Model file for the job. Use its own axes, mm. A direction names the side the tool comes from. Round coordinates to 2 decimals unless told otherwise and drop trailing zeros. Loops run counter-clockwise (first coordinate to the right, second up) from the corner with the lowest first, then second, coordinate; pieces in that order, holes last. Notation, with made-up numbers: M 18,47 L 48,47 A33 ccw 48,83 Z; hole C 81.5,14 d11. An arc over 180 degrees is marked long. Use a Markdown table: item, result. Add a question column.
Q1. Cut at D-D (z = -72.9). Give the cut face in (x, y), plus the area to 3 significant figures.
Q2. Tool access for faces 1 (the face through (43, 2.8, -34)), 2 (the face through (8.8, 2, -61)), 3 (the face through (38, 3, -71)), 4 (the face through (45, 2, -56)), 5 (the face through (26.2, 2, -73)): list every direction of +Z, -Z, +X, -X, +Y, -Y with a clear straight run to the whole face (end or side of a thin tool).
Q3. Cut at A-A (x = 37.5). Give the cut face in (y, z).
Q4. Pin check, flat tips, straight feed: pin 1 (0.8 mm diameter, centred on y = 2, z = -44, fed in from +X); pin 2 (1.5 mm diameter, centred on y = 1.5, z = -58.5, fed in from +X); pin 3 (2 mm diameter, centred on y = 1.5, z = -20.5, fed in from -X). Stop position of each tip, or through.
Q5. Probe line 1 (X direction, y = 0.85, z = -50); line 2 (Z direction, x = 25, y = 1.1); line 3 (Z direction, x = 8, y = 2.85). List the from-to ranges inside material, lowest first. Write a range as from..to.
Q6. Cut at C-C (x = 21). Give the cut face in (y, z), plus the area to 3 significant figures.
Q7. Cut at B-B (z = -44). Give the cut face in (x, y).
Q8. Mould opens along Z. For faces 6 (the face through (-3, 2, -17)), 7 (the face through (2, 0, -41)), 8 (the face through (23, 2, -69.8)), 9 (the face through (10, 1, -67.4)) say: +Z half, -Z half, draft (parallel to the pull), parting line (faces both ways), or undercut.
from build123d import *

# Parameters (mm, degrees)
SKETCH_1_W           = 50
SKETCH_1_H           = 76
EXTRUDE_1_DEPTH      = 4
EXTRUDE_2_DEPTH      = 4
SKETCH_4_W           = 6.4
SKETCH_4_H           = 6.2
CUT_EXTRUDE_1_DEPTH  = 4
CHAMFER_1_SIZE       = 3
SKETCH_6_W           = 2
SKETCH_6_H           = 30
CUT_EXTRUDE_3_DEPTH  = 5
SKETCH_7_W           = 28.1
SKETCH_7_H           = 63.9
CUT_EXTRUDE_4_DEPTH  = 1.2
CUT_EXTRUDE_5_DEPTH  = 3.8
CUT_EXTRUDE_6_DEPTH  = 0.8
SKETCH_10_R          = 0.85
CUT_EXTRUDE_7_DEPTH  = 3
SKETCH_11_R          = 1.5
CUT_EXTRUDE_8_DEPTH  = 5
CHAMFER_2_SIZE       = 1
SKETCH_12_W          = 7
SKETCH_12_H          = 10.1
CUT_EXTRUDE_9_DEPTH  = 3
CHAMFER_3_SIZE       = 0.2
CUT_EXTRUDE_10_DEPTH = 2


with BuildPart() as part:
    # 草图1 → 凸台-拉伸1 (new body)
    with BuildSketch(Plane(origin=(0, 0, 0), x_dir=(1, 0, 0), z_dir=(0, 1, 0))):
        with Locations((25, 38)):
            Rectangle(SKETCH_1_W, SKETCH_1_H)
    extrude(amount=EXTRUDE_1_DEPTH)

    # 草图3 → 凸台-拉伸2 (add)
    with BuildSketch(Plane(origin=(0, 4, 0), x_dir=(1, 0, 0), z_dir=(0, 1, 0))):
        Polygon((0, 0), (-5, 5), (-5, 15), (0, 20), align=None)
        Polygon((0, 30), (-4, 34), (-4, 66), (0, 70), align=None)
    extrude(amount=-EXTRUDE_2_DEPTH)

    # 草图4 → 切除-拉伸1 (cut)
    with BuildSketch(Plane(origin=(0, 4, 0), x_dir=(1, 0, 0), z_dir=(0, 1, 0))):
        with Locations((23, 72.9)):
            Rectangle(SKETCH_4_W, SKETCH_4_H)
    extrude(amount=-CUT_EXTRUDE_1_DEPTH, mode=Mode.SUBTRACT)

    # 倒角1
    chamfer_1_edges = [part.edges().sort_by_distance(p)[0] for p in [
        (50, 2, 0),
    ]]
    chamfer(chamfer_1_edges, length=CHAMFER_1_SIZE)

    # 草图6 → 切除-拉伸3 (cut, through all)
    with BuildSketch(Plane(origin=(0, 4, 0), x_dir=(1, 0, 0), z_dir=(0, 1, 0))):
        with Locations((49, 50)):
            Rectangle(SKETCH_6_W, SKETCH_6_H)
    extrude(amount=-CUT_EXTRUDE_3_DEPTH, mode=Mode.SUBTRACT)

    # 草图7 → 切除-拉伸4 (cut)
    with BuildSketch(Plane(origin=(0, 4, 0), x_dir=(1, 0, 0), z_dir=(0, 1, 0))):
        with Locations((29.95, 33.95)):
            Rectangle(SKETCH_7_W, SKETCH_7_H)
    extrude(amount=-CUT_EXTRUDE_4_DEPTH, mode=Mode.SUBTRACT)

    # 草图8 → 切除-拉伸5 (cut, through all)
    with BuildSketch(Plane(origin=(0, 2.8, 0), x_dir=(1, 0, 0), z_dir=(0, 1, 0))):
        Polygon((41.6, 65.9), (41.6, 2), (18.3, 2), (18.3, 25), (29.3, 25), (29.3, 30), (18.3, 30), (18.3, 65.9), align=None)
    extrude(amount=-CUT_EXTRUDE_5_DEPTH, mode=Mode.SUBTRACT)

    # 草图9 → 切除-拉伸6 (cut)
    with BuildSketch(Plane.XZ):
        Polygon((18.3, -25), (18.3, -9), (2.4, -9), (2.4, -61), (4.4, -61), (4.4, -62.5), (5.8, -62.5), (5.8, -67.4), (15.2, -67.4), (15.2, -62.5), (18.3, -62.5), (18.3, -30), (29.3, -30), (29.3, -25), align=None)
    extrude(amount=-CUT_EXTRUDE_6_DEPTH, mode=Mode.SUBTRACT)

    # 草图10 → 切除-拉伸7 (cut)
    with BuildSketch(Plane(origin=(48, 0, 0), x_dir=(0, 0, -1), z_dir=(1, 0, 0))):
        with Locations((44, 2)):
            Circle(SKETCH_10_R)
        with Locations((56, 2)):
            Circle(SKETCH_10_R)
    extrude(amount=-CUT_EXTRUDE_7_DEPTH, mode=Mode.SUBTRACT)

    # 草图11 → 切除-拉伸8 (cut, through all)
    with BuildSketch(Plane(origin=(0, 4, 0), x_dir=(1, 0, 0), z_dir=(0, 1, 0))):
        with Locations((-0.9, 50)):
            Circle(SKETCH_11_R)
        with Locations((31, 72.9)):
            Circle(SKETCH_11_R)
        with Locations((8, 3.05)):
            Circle(SKETCH_11_R)
        with Locations((47, 21)):
            Circle(SKETCH_11_R)
    extrude(amount=-CUT_EXTRUDE_8_DEPTH, mode=Mode.SUBTRACT)

    # 倒角2
    chamfer_2_edges = [part.edges().sort_by_distance(p)[0] for p in [
        (50, 2, -65),
        (50, 2, -35),
    ]]
    chamfer(chamfer_2_edges, length=CHAMFER_2_SIZE)

    # 草图12 → 切除-拉伸9 (cut)
    with BuildSketch(Plane.XZ):
        with Locations((38.1, -70.95)):
            Rectangle(SKETCH_12_W, SKETCH_12_H)
    extrude(amount=-CUT_EXTRUDE_9_DEPTH, mode=Mode.SUBTRACT)

    # 倒角3
    chamfer_3_edges = [part.edges().sort_by_distance(p)[0] for p in [
        (26.2, 2, -76),
        (45.8, 0, -76),
        (50, 2, -76),
        (38.1, 4, -76),
    ]]
    chamfer(chamfer_3_edges, length=CHAMFER_3_SIZE)

    # 草图13 → 切除-拉伸10 (cut)
    with BuildSketch(Plane.XZ.offset(-0.8)):
        Polygon((5.8, -67.4), (15.2, -67.4), (15.2, -65.4), (12.2, -65.4), (12.2, -59.9), (18.3, -59.9), (18.3, -56.9), (8.8, -56.9), (8.8, -59.955757414), (8.8, -65.4), (5.8, -65.4), align=None)
    extrude(amount=-CUT_EXTRUDE_10_DEPTH, mode=Mode.SUBTRACT)


solid = part.part
Checked values:
| question | item | result |
|---|---|---|
| 1 | outline | M 0,0 L 19.8,0 L 19.8,4 L 0,4 Z; M 26.2,0 L 29.5,0 L 29.5,4 L 26.2,4 Z; M 32.5,0 L 34.6,0 L 34.6,3 L 41.6,3 L 41.6,0 L 50,0 L 50,4 L 32.5,4 Z |
| 1 | area | 141 mm^2 |
| 2 | face 1 | +Y |
| 2 | face 2 | -Y |
| 2 | face 3 | -Z, -Y |
| 2 | face 4 | +X |
| 2 | face 5 | -Z, +Y, -Y |
| 3 | outline | M 0,-2 L 4,-2 L 4,0 L 0,0 Z; M 3,-76 L 3.8,-76 L 4,-75.8 L 4,-65.9 L 3,-65.9 Z |
| 4 | pin 1 | stops at x = 45 |
| 4 | pin 2 | stops at x = 48 |
| 4 | pin 3 | stops at x = -0.5 |
| 5 | line 1 | x = -4..-2.4, 0.6..18.3, 41.6..48 |
| 5 | line 2 | z = -69.8..-65.9, -30..-25, -2..0 |
| 5 | line 3 | z = -76..-4.55, -1.55..0 |
| 6 | outline | M 0,-69.8 L 4,-69.8 L 4,-65.9 L 0,-65.9 Z; M 0,-2 L 4,-2 L 4,0 L 0,0 Z; M 0.8,-30 L 2.8,-30 L 2.8,-25 L 0.8,-25 Z |
| 6 | area | 33.6 mm^2 |
| 7 | outline | M -4,0 L 2.4,0 L 2.4,0.8 L 18.3,0.8 L 18.3,2.8 L 15.9,2.8 L 15.9,4 L -4,4 Z; M 41.6,0 L 48,0 L 48,1.15 L 45,1.15 L 45,2.85 L 48,2.85 L 48,4 L 44,4 L 44,2.8 L 41.6,2.8 Z |
| 8 | face 6 | undercut |
| 8 | face 7 | draft |
| 8 | face 8 | -Z half |
| 8 | face 9 | undercut |
